For this review, take the finished solid that the model builds, in its own axes (mm). A direction names the side the tool comes from. Coordinates: 2 decimals unless noted, no trailing zeros. Loops run counter-clockwise (first coordinate to the right, second up) from the corner with the lowest first, then second, coordinate; pieces in that order, holes last. Notation, with made-up numbers: (68, -4) - (83, -4) arc R20 ccw to (83, 30) - close; hole circle Ø4 at (65, 9.5). An arc over 180 degrees is marked (long way). Answer as a JSON object with one key per item and string values. Group by question number.
Item 1: To check wall thickness, follow line 1 (Y direction, x = 0, z = 1); line 2 (X direction, y = -10.5, z = 3); line 3 (Y direction, x = -7, z = 1). State the ranges of each line that lie inside material, in increasing order.
Item 2: We need section C-C (z = 12.5). Give the boundary of the cut face in (x, y).
Item 3: We need section D-D (y = -7.75). Give the boundary of the cut face in (x, z), then the cut area to 3 significant figures.
Item 4: Mouldability with a two-part tool opening along Y and no side actions: class faces 3 (the cylindrical face through (-8.5, 0.07, 1.01)), 4 (the flat face through (-28, -3, 32)), 5 (the flat face through (0, -12.5, 1)) as released by +Y, released by -Y, zero draft, split by the parting line, or undercut.
Item 5: We need section A-A (z = 45). Give the boundary of the cut face in (x, y).
Item 6: Tool access review of faces 1 (the cylindrical face through (-27, 6.1, 53.2)), 2 (the flat face through (-26, -3, 33)): name each direction out of +Z, -Z, +X, -X, +Y, -Y from which nothing blocks a thin tool from reaching the whole face with its end or side.
Item 7: We need section B-B (x = -7). Give the boundary of the cut face in (y, z), then the cut area to 3 significant figures.
Item 8: Clearance check with flat-ended pins moving along their axes: pin 1 (3 mm diameter, centred on x = -1.5, y = 3, fed in from +Z); pin 2 (1.8 mm diameter, centred on y = 0, z = 45, fed in from -X). State where each tip first meets the part, or that it passes through.
from build123d import *

# Parameters (mm, degrees)
SKETCH_1_W          = 56
SKETCH_1_H          = 25
EXTRUDE_1_DEPTH     = 64.5
CUT_EXTRUDE_1_DEPTH = 75.627407834
SKETCH_4_R          = 4
SKETCH_4_R_2        = 1.5
CUT_EXTRUDE_3_DEPTH = 70.616808315
CUT_EXTRUDE_4_DEPTH = 87.327863405
SKETCH_5_R          = 4
SKETCH_5_R_2        = 1.5
CUT_EXTRUDE_5_DEPTH = 87.327863405


with BuildPart() as part:
    # 草图1 → 凸台-拉伸1 (new body)
    with BuildSketch(Plane.XY):
        Rectangle(SKETCH_1_W, SKETCH_1_H)
    extrude(amount=EXTRUDE_1_DEPTH)

    # 草图2 → 切除-拉伸1 (cut, through all)
    with BuildSketch(Plane.XZ.offset(12.5)):
        Polygon((0, 64.5), (26, 64.5), (26, 2), (-26, 2), (-26, 64.5), align=None)
    extrude(amount=-CUT_EXTRUDE_1_DEPTH, mode=Mode.SUBTRACT)

    # 草图4 → 切除-拉伸3 (cut, through all)
    with BuildSketch(Plane.XY.offset(2)):
        Circle(SKETCH_4_R)
        with Locations((0, 7)):
            Circle(SKETCH_4_R_2)
        with Locations((0, -7)):
            Circle(SKETCH_4_R_2)
        with Locations((-7, 0)):
            Circle(SKETCH_4_R_2)
        with Locations((7, 0)):
            Circle(SKETCH_4_R_2)
        with Locations((18.6, 0)):
            Circle(SKETCH_4_R_2)
        with Locations(Location((-18.6, 0, 0), (0, 0, 180))):
            Circle(SKETCH_4_R_2)
    extrude(amount=-CUT_EXTRUDE_3_DEPTH, mode=Mode.SUBTRACT)

    # 草图3 → 切除-拉伸4 (cut, through all)
    with BuildSketch(Plane(origin=(28, 0, 0), x_dir=(0, 0, -1), z_dir=(1, 0, 0))):
        with BuildLine():
            ThreePointArc((-64.5, 0), (-60.838834765, 8.838834765), (-52, 12.5))
            Line((-52, 12.5), (-64.5, 12.5))
            Line((-64.5, 12.5), (-64.5, 0))
        make_face()
        with BuildLine():
            ThreePointArc((-52, -12.5), (-60.838834765, -8.838834765), (-64.5, 0))
            Line((-64.5, 0), (-64.5, -12.5))
            Line((-64.5, -12.5), (-52, -12.5))
        make_face()
    extrude(amount=-CUT_EXTRUDE_4_DEPTH, mode=Mode.SUBTRACT)

    # 草图5 → 切除-拉伸5 (cut, through all)
    with BuildSketch(Plane(origin=(28, 0, 0), x_dir=(0, 0, -1), z_dir=(1, 0, 0))):
        with Locations((-52, 0)):
            Circle(SKETCH_5_R)
        with Locations((-52, 7)):
            Circle(SKETCH_5_R_2)
        with Locations((-59, 0)):
            Circle(SKETCH_5_R_2)
        with Locations((-52, -7)):
            Circle(SKETCH_5_R_2)
        with Locations((-45, 0)):
            Circle(SKETCH_5_R_2)
        with Locations((-33.4, 0)):
            Circle(SKETCH_5_R_2)
        with Locations((-16.5, 0)):
            Circle(SKETCH_5_R_2)
    extrude(amount=-CUT_EXTRUDE_5_DEPTH, mode=Mode.SUBTRACT)


solid = part.part
Check sheet entries:
{
 "1": {"line 1": "y = -12.5 to -8.5, -5.5 to -4, 4 to 5.5, 8.5 to 12.5", "line 2": "x = -28 to -26, 26 to 28", "line 3": "y = -12.5 to -1.5, 1.5 to 12.5"},
 "2": {"outline": "(-28, -12.5) - (-26, -12.5) - (-26, 12.5) - (-28, 12.5) - close; (26, -12.5) - (28, -12.5) - (28, 12.5) - (26, 12.5) - close"},
 "3": {"outline": "(-28, 0) - (-1.3, 0) - (-1.3, 2) - (-26, 2) - (-26, 50.7) - (-28, 50.7) - close; (-28, 53.3) - (-26, 53.3) - (-26, 61.81) - (-28, 61.81) - close; (1.3, 0) - (28, 0) - (28, 50.7) - (26, 50.7) - (26, 2) - (1.3, 2) - close; (26, 53.3) - (28, 53.3) - (28, 61.81) - (26, 61.81) - close", "area": "336 mm2"},
 "4": {"face 3": "undercut", "face 4": "zero draft", "face 5": "released by -Y"},
 "5": {"outline": "(-28, -12.5) - (-26, -12.5) - (-26, -1.5) - (-28, -1.5) - close; (-28, 1.5) - (-26, 1.5) - (-26, 12.5) - (-28, 12.5) - close; (26, -12.5) - (28, -12.5) - (28, -1.5) - (26, -1.5) - close; (26, 1.5) - (28, 1.5) - (28, 12.5) - (26, 12.5) - close"},
 "6": {"face 1": "+X, -X", "face 2": "+Z, +Y, -Y"},
 "7": {"outline": "(-12.5, 0) - (-1.5, 0) - (-1.5, 2) - (-12.5, 2) - close; (1.5, 0) - (12.5, 0) - (12.5, 2) - (1.5, 2) - close", "area": "44.0 mm2"},
 "8": {"pin 1": "stops at z = 2", "pin 2": "passes through"}
}
